Read the model definition and answer for the solid it produces. Units are mm, in the model's axes. Coordinates: 2 decimals unless noted, no trailing zeros. Write each loop counter-clockwise with the first axis right and the second up, starting at its lowest first coordinate (ties: lowest second). Pieces come first, ordered by that corner, then holes. Notation, with made-up numbers: (19, 8) -> (73, 8) arc R21 ccw to (73, 17) -> close; hole circle Ø5 at (-18, 45). An arc over 180 degrees is marked (long way). Answer in a Markdown table with one row per item. Add a question column.
Item 1: Given pin 1 Ø6 at (y, z) = (-8, 32) entering from -X; pin 2 Ø2 at (x, z) = (7.5, 16) entering from +Y; pin 3 Ø12 at (x, z) = (6.5, 9) entering from +Y, each flat-ended and moving along its own axis, determine where each tip first touches the part or whether it passes through.
Item 2: Straight lines are drawn through the part: line 1 (Z direction, x = 5, y = 6.5); line 2 (Z direction, x = -9.5, y = -4); line 3 (X direction, y = -5.5, z = -2). For each, find the intervals that lie inside material, in ascending order. Write a range as from..to.
Item 3: Section A-A on z = 8 is taken. Write down the section's boundary in (x, y), then the cut area to 3 significant figures.
```python
from build123d import *

# Parameters (mm, degrees)
F2_R = 2
F3_R = 7


with BuildPart() as f1:
    # F0 (on Front) → F1 (revolve)
    with BuildSketch(Plane.XZ):
        with BuildLine():
            Line((15, 0), (15, 20))
            add(Edge.make_bspline(
                [(15, 20), (14.5080885538, 22.063984506), (13.9999463782, 37.4930197538), (10.6078177215, 48.1757262572), (7.7037410613, 54.3763197541), (5.6345020381, 57.6882536536), (2.5841033515, 60), (0, 60)],
                knots=[0, 0, 0, 0, 0.2796626362, 0.525434394, 0.6977638983, 0.8311479045, 1, 1, 1, 1], degree=3))
            Line((0, 60), (0, -25))
            Line((0, -25), (15, -25))
            Line((15, -25), (15, -15))
            ThreePointArc((15, -15), (7.5, -7.5), (15, 0))
        make_face()
    revolve(axis=Axis((0, 0, 9.3989223242), (0, 0, -1)))

    # F2
    f2_edges = [f1.edges().sort_by_distance(p)[0] for p in [
        (-15, 0, -15),
        (-15, 0, -25),
    ]]
    fillet(f2_edges, radius=F2_R)

    # F3
    f3_edges = [f1.edges().sort_by_distance(p)[0] for p in [
        (-15, 0, 0),
    ]]
    fillet(f3_edges, radius=F3_R)


solid = f1.part
```
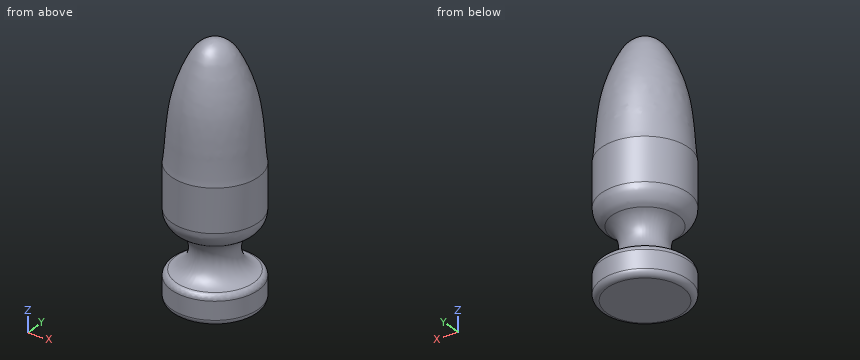
Results below:
| question | item | result |
|---|---|---|
| 1 | pin 1 | stops at x = -12.99 |
| 1 | pin 2 | stops at y = 13.52 |
| 1 | pin 3 | stops at y = 14.99 |
| 2 | line 1 | z = -25..-10.67, -4.33..53.21 |
| 2 | line 2 | z = -25..-13.35, -1.65..48.42 |
| 2 | line 3 | x = -8.23..8.23 |
| 3 | outline | circle Ø30 at (0, 0) |
| 3 | area | 707 mm2 |
